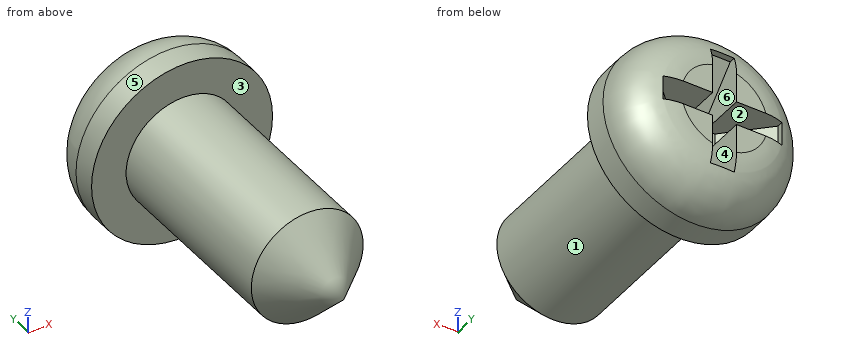
```python
from build123d import *

# Parameters (mm, degrees)
CUT_EXTRUDE1_DEPTH = 1
CHAMFER1_SIZE      = 0.8


with BuildPart() as part:
    # Sketch1 → Revolve1 (revolve)
    with BuildSketch(Plane.XY):
        with BuildLine():
            Line((1.175, 0), (1.9, 0))
            Line((1.9, 0), (1.9, 0.5))
            ThreePointArc((1.9, 0.5), (1.607106781, 1.207106781), (0.9, 1.5))
            Line((0.9, 1.5), (0, 1.5))
            Line((0, 1.5), (0, -5.2))
            Line((0, -5.2), (1.175, -4.025))
            Line((1.175, -4.025), (1.175, 0))
        make_face()
    revolve(axis=Axis((0, -5.2, 0), (0, -1, 0)))

    # Sketch2 → Cut-Extrude1 (cut)
    with BuildSketch(Plane(origin=(0, 1.5, 0), x_dir=(1, 0, 0), z_dir=(0, 1, 0))):
        Polygon((0.25, 0.25), (1.25, 0.25), (1.25, -0.25), (0.25, -0.25), (0.25, -1.25), (-0.25, -1.25), (-0.25, -0.25), (-1.25, -0.25), (-1.25, 0.25), (-0.25, 0.25), (-0.25, 1.25), (0.25, 1.25), align=None)
    extrude(amount=-CUT_EXTRUDE1_DEPTH, mode=Mode.SUBTRACT)

    # Chamfer1
    chamfer1_edges = [part.edges().sort_by_distance(p)[0] for p in [
        (-1.25, 0.5, 0),
        (0, 0.5, -1.25),
        (1.25, 0.5, 0),
        (0, 0.5, 1.25),
    ]]
    chamfer(chamfer1_edges, length=CHAMFER1_SIZE)


solid = part.part
```
Here's how the part is built. I have some questions about the finished solid (model axes, mm). Face numbers are marked on the shaded views. A direction names the side the tool comes from. Give positions to 0.01 mm unless a question says otherwise; leave off trailing zeros. Loops run counter-clockwise (first coordinate to the right, second up) from the corner with the lowest first, then second, coordinate; pieces in that order, holes last. Notation, with made-up numbers: M -0.75,66.25 L 32.25,66.25 A23 ccw 32.25,94.25 Z; hole C -3.5,56 d2. An arc over 180 degrees is marked long. Put each result on its own line as item: value. Start each with the question number.
(1) Will these pins go through, and if not, where does the flat tip stop? pin 1 Ø2 at (y, z) = (-4, 0) entering from +X (3 decimals); pin 2 Ø0.8 at (x, y) = (-1, 1) entering from +Z; pin 3 Ø0.5 at (y, z) = (1, 1) entering from +X.
(2) For the marked faces 1 and 2, which set-ups out of +Z, -Z, +X, -X, +Y, -Y let a thin tool reach every point of the face, with its end or its side?
(3) I want a section at A-A on y = -2.5. Please give me the cut outline in (x, z) (3 decimals).
(4) I need wall thicknesses on line 1 along Z through (x, y) = (0.65, -2.75); line 2 along X through (y, z) = (-4, -0.75); line 3 along Y through (x, z) = (-1.35, -1.1). Which ranges of each line are inside material? Lowest first, please. Write a range as [from, to].
(5) If we mould it in two halves opening along Z, with no side actions, what happens to the marked faces 3, 4, 5 and 6? For each: +Z half, -Z half, draft (parallel to the pull), parting line (faces both ways), or undercut.
Answer block:
1. pin 1: x = 1.175
1. pin 2: z = 1.74
1. pin 3: x = 1.65
2. face 1: -Y
2. face 2: +Y
3. outline: C 0,0 d2.35
4. line 1: [-0.98, 0.98]
4. line 2: [-0.9, 0.9]
4. line 3: [0, 1.04]
5. face 3: draft
5. face 4: undercut
5. face 5: parting line
5. face 6: undercut
